```python
from build123d import *

# Parameters (mm, degrees)
SKETCH1_W           = 35.3568
SKETCH1_H           = 31.3309
SKETCH1_R           = 1.524
BOSS_EXTRUDE1_DEPTH = 1.5875
SKETCH2_W           = 2.4638
SKETCH2_H           = 9.9568
SKETCH2_W_2         = 9.9568
SKETCH2_H_2         = 2.4638
BOSS_EXTRUDE2_DEPTH = 2.4384
SKETCH3_W           = 10.033
SKETCH3_H           = 20.32
BOSS_EXTRUDE3_DEPTH = 8.0899
SKETCH4_W           = 5.9436
SKETCH4_H           = 14.9352
BOSS_EXTRUDE4_DEPTH = 7.1628
SKETCH5_R           = 1.4605
BOSS_EXTRUDE5_DEPTH = 5.1562


with BuildPart() as part:
    # Sketch1 → Boss-Extrude1 (new body)
    with BuildSketch(Plane(origin=(0, 0, 0), x_dir=(1, 0, 0), z_dir=(0, 1, 0))):
        Rectangle(SKETCH1_W, SKETCH1_H)
        with Locations((14.9352, -13.10005)):
            Circle(SKETCH1_R, mode=Mode.SUBTRACT)
        with Locations((14.9352, 13.10005)):
            Circle(SKETCH1_R, mode=Mode.SUBTRACT)
        with Locations((-14.9352, -13.10005)):
            Circle(SKETCH1_R, mode=Mode.SUBTRACT)
        with Locations((-14.9352, 13.10005)):
            Circle(SKETCH1_R, mode=Mode.SUBTRACT)
    extrude(amount=BOSS_EXTRUDE1_DEPTH)

    # Sketch2 → Boss-Extrude2 (add)
    with BuildSketch(Plane(origin=(0, 1.5875, 0), x_dir=(1, 0, 0), z_dir=(0, 1, 0))):
        with Locations((-10.9347, 5.31495)):
            Rectangle(SKETCH2_W, SKETCH2_H)
        with Locations((-4.1021, -10.24255)):
            Rectangle(SKETCH2_W_2, SKETCH2_H_2)
    extrude(amount=BOSS_EXTRUDE2_DEPTH)

    # Sketch3 → Boss-Extrude3 (add)
    with BuildSketch(Plane(origin=(0, 1.5875, 0), x_dir=(1, 0, 0), z_dir=(0, 1, 0))):
        with Locations((-3.7465, 4.38785)):
            Rectangle(SKETCH3_W, SKETCH3_H)
    extrude(amount=BOSS_EXTRUDE3_DEPTH)

    # Sketch4 → Boss-Extrude4 (add)
    with BuildSketch(Plane(origin=(0, 1.5875, 0), x_dir=(1, 0, 0), z_dir=(0, 1, 0))):
        with Locations((4.826, 5.86105)):
            Rectangle(SKETCH4_W, SKETCH4_H)
    extrude(amount=BOSS_EXTRUDE4_DEPTH)

    # Sketch5 → Boss-Extrude5 (add)
    with BuildSketch(Plane(origin=(0, 1.5875, 0), x_dir=(1, 0, 0), z_dir=(0, 1, 0))):
        with Locations((12.7635, 9.30275)):
            Circle(SKETCH5_R)
        with Locations((12.7635, 5.01015)):
            Circle(SKETCH5_R)
        with Locations((12.7635, 0.71755)):
            Circle(SKETCH5_R)
        with Locations((12.7635, -3.57505)):
            Circle(SKETCH5_R)
    extrude(amount=BOSS_EXTRUDE5_DEPTH)


solid = part.part
```
Model file for the job. Use its own axes, mm. A direction names the side the tool comes from. Give positions to 0.01 mm unless a question says otherwise; leave off trailing zeros. Loops run counter-clockwise (first coordinate to the right, second up) from the corner with the lowest first, then second, coordinate; pieces in that order, holes last. Notation, with made-up numbers: M 53.5,-6.5 L 111.5,-6.5 A20 cw 111.5,27.5 Z; hole C 76.25,62 d5. An arc over 180 degrees is marked long. Use one line per item in the form item = value.
Item 1: Slice it at B-B on x = 7. List the corners of the cut face in (y, z).
Filled in:
outline = M 0,-15.67 L 1.59,-15.67 L 1.59,-13.33 L 8.75,-13.33 L 8.75,1.61 L 1.59,1.61 L 1.59,15.67 L 0,15.67 Z
Item 2: Drill centre lines: L1, parallel to Z at x = -0.5, y = 3.75; L2, parallel to X at y = 5.75, z = -6; L3, parallel to X at y = 2.75, z = -1.5. Where is each one in solid material? Low to high.
Filled in:
L1 = -14.55 to 5.77, 9.01 to 11.47
L2 = -8.76 to 1.27, 1.85 to 7.8, 11.69 to 13.84
L3 = -12.17 to -9.7, -8.76 to 1.27, 1.85 to 7.8, 11.53 to 14
Item 3: Two-plate mould, pull along X, no slides. Class faces 1 (the flat face through (13, 6.744, 4)), 2 (the flat face through (7.798, 5, -6)), 3 (the flat face through (-12.167, 3, -5)): released by +X, released by -X, zero draft, split by the parting line, or undercut.
Filled in:
face_1 = zero draft
face_2 = undercut
face_3 = released by -X
Item 4: Slice it at C-C on z = -12.5. List the corners of the cut face in (x, y), and give its area (3 significant figures).
Filled in:
outline = M -17.68,0 L -16.34,0 L -16.34,1.59 L -17.68,1.59 Z; M -13.53,0 L 13.53,0 L 13.53,1.59 L 7.8,1.59 L 7.8,8.75 L 1.85,8.75 L 1.85,1.59 L 1.27,1.59 L 1.27,9.68 L -8.76,9.68 L -8.76,1.59 L -13.53,1.59 Z; M 16.34,0 L 17.68,0 L 17.68,1.59 L 16.34,1.59 Z
area = 171 mm^2
Item 5: Which spindle directions (+Z, -Z, +X, -X, +Y, -Y) get a long thin tool onto all of the face, cutting with end or side? Do faces 4 (the flat face through (-11, 3, -0.337)), 5 (the flat face through (-4, 6, -14.548)), 6 (the flat face through (13, 6.744, -1)), 7 (the flat face through (5, 5, -13.329)). Say none if no direction does.
Filled in:
face_4 = +Z, -X, +Y
face_5 = -Z, +X, -X, +Y
face_6 = +Z, -Z, +X, +Y
face_7 = -Z, +X, +Y
Item 6: Slice it at A-A on y = 8.25. List the corners of the cut face in (x, z), and give its area (3 significant figures).
Filled in:
outline = M -8.76,-14.55 L 1.27,-14.55 L 1.27,5.77 L -8.76,5.77 Z; M 1.85,-13.33 L 7.8,-13.33 L 7.8,1.61 L 1.85,1.61 Z
area = 293 mm^2
Item 7: Slice it at D-D on z = -7. List the corners of the cut face in (x, y).
Filled in:
outline = M -17.68,0 L 17.68,0 L 17.68,1.59 L 7.8,1.59 L 7.8,8.75 L 1.85,8.75 L 1.85,1.59 L 1.27,1.59 L 1.27,9.68 L -8.76,9.68 L -8.76,1.59 L -9.7,1.59 L -9.7,4.03 L -12.17,4.03 L -12.17,1.59 L -17.68,1.59 Z
Item 8: Flat gauge pins, fed straight in: pin 1 Ø0.7 at (y, z) = (2.5, -7.5) entering from -X; pin 2 Ø2.5 at (x, z) = (12.5, 3.5) entering from +Y; pin 3 Ø0.7 at (x, z) = (-5, 10.5) entering from +Y; pin 4 Ø1.5 at (y, z) = (8.5, 8) entering from +X. Where does each tip first touch, or does it go through?
Filled in:
pin_1 = -12.17
pin_2 = 6.74
pin_3 = 4.03
pin_4 = through
